from build123d import *

# Parameters (mm, degrees)
F0_R     = 14
F0_R_2   = 1.1
F1_DEPTH = 3
F2_R     = 6
F3_DEPTH = 10
F5_DEPTH = 13.001
F6_R     = 0.875
F7_DEPTH = 14.001
F8_R     = 0.875
F9_DEPTH = 14.001


with BuildPart() as f1:
    # F0 (on Front) → F1 (new body)
    with BuildSketch(Plane.XZ):
        Circle(F0_R)
        with Locations((-8.660254, -5)):
            Circle(F0_R_2, mode=Mode.SUBTRACT)
        with Locations((8.660254, -5)):
            Circle(F0_R_2, mode=Mode.SUBTRACT)
        with Locations((0, 10)):
            Circle(F0_R_2, mode=Mode.SUBTRACT)
    extrude(amount=F1_DEPTH)

    # F2 (on face) → F3 (join)
    with BuildSketch(Plane.XZ.offset(3)):
        Circle(F2_R)
    extrude(amount=F3_DEPTH)

    # F4 (on face) → F5 (cut, through all)
    with BuildSketch(Plane.XZ.offset(13)):
        with BuildLine():
            Line((1.5, 1.322876), (-1.5, 1.322876))
            ThreePointArc((-1.5, 1.322876), (0, -2), (1.5, 1.322876))
        make_face()
    extrude(amount=-F5_DEPTH, mode=Mode.SUBTRACT)

    # F6 (on Top) → F7 (cut, through all)
    with BuildSketch(Plane.XY):
        with Locations((0, -9)):
            Circle(F6_R)
    extrude(amount=F7_DEPTH, mode=Mode.SUBTRACT)

    # F8 (on Right) → F9 (cut, through all)
    with BuildSketch(Plane.YZ):
        with Locations((-9, 0)):
            Circle(F8_R)
    extrude(amount=F9_DEPTH, mode=Mode.SUBTRACT)


solid = f1.part
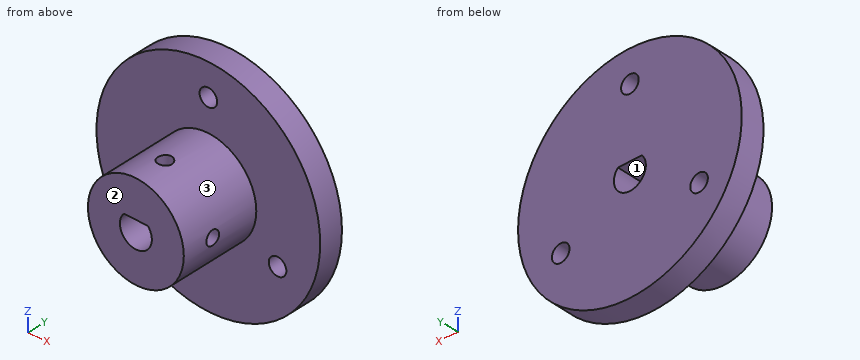
Model file for the job. Use its own axes, mm. Face numbers are marked on the shaded views. A direction names the side the tool comes from. Give positions to 0.01 mm unless a question says otherwise; leave off trailing zeros. Loops run counter-clockwise (first coordinate to the right, second up) from the corner with the lowest first, then second, coordinate; pieces in that order, holes last.
Item 1: Slice it at C-C (z = 10). Write the cut outline in (x, y), plus the area to 3 significant figures.
Check values:
outline: (-9.8, -3) - (-1.1, -3) - (-1.1, 0) - (-9.8, 0) - close; (1.1, -3) - (9.8, -3) - (9.8, 0) - (1.1, 0) - close
area: 52.2 mm2
Item 2: Which spindle directions (+Z, -Z, +X, -X, +Y, -Y) get a long thin tool onto all of the face, cutting with end or side? Do the marked faces 1, 2 and 3. Say none if no direction does.
Check values:
face 1: +Y, -Y
face 2: +Z, -Z, +X, -X, -Y
face 3: -Y
Item 3: Slice it at D-D (y = -6.5). Write the cut outline in (x, z).
Check values:
outline: circle Ø12 at (0, 0); hole (-1.5, 1.32) arc R2 ccw (long way) to (1.5, 1.32) - close
Item 4: Drop flat-ended pins along their axis: P1, Ø2.5, axis at x = 0, z = 0, coming from the +Y side; P2, Ø6, axis at x = 8, z = 10.5, coming from the -Y side; P3, Ø10, axis at x = -5.5, z = 3, coming from the -Y side; P4, Ø2, axis at x = 2, y = -5, coming from the +Z side. Give the stop position or say it passes through.
Check values:
P1: passes through
P2: stops at y = -3
P3: stops at y = -13
P4: stops at z = 5.92
Item 5: Slice it at B-B (y = -1.75). Write the cut outline in (x, z).
Check values:
outline: circle Ø28 at (0, 0); hole circle Ø2.2 at (-8.66, -5); hole (-1.5, 1.32) arc R2 ccw (long way) to (1.5, 1.32) - close; hole circle Ø2.2 at (0, 10); hole circle Ø2.2 at (8.66, -5)
Item 6: Slice it at A-A (z = 0). Write the cut outline in (x, y) (3 decimals).
Check values:
outline: (-14, -3) - (-6, -3) - (-6, -13) - (-2, -13) - (-2, 0) - (-14, 0) - close; (2, -13) - (6, -13) - (6, -9.875) - (2, -9.875) - close; (2, -8.125) - (6, -8.125) - (6, -3) - (14, -3) - (14, 0) - (2, 0) - close
Item 7: Drill centre lines: line 1 along Z through (x, y) = (0, -8.75); line 2 along Y through (x, z) = (5, 12.5); line 3 along Z through (x, y) = (-0.5, -4.5). Where is each one in solid material? Low to high.
Check values:
line 1: z = -6 to -2
line 2: y = -3 to 0
line 3: z = -5.98 to -1.94, 1.32 to 5.98
